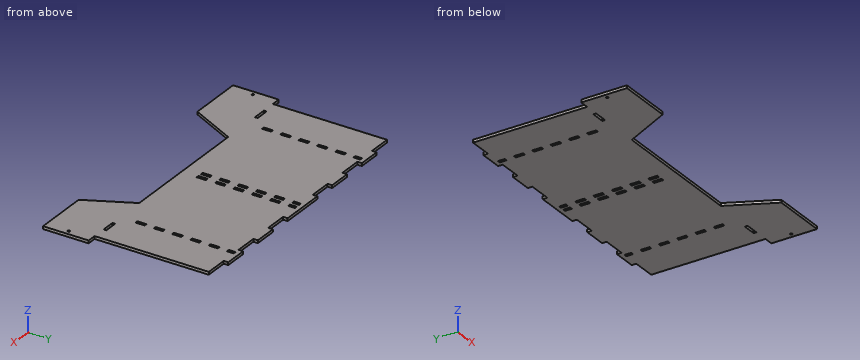
```python
from build123d import *

# Parameters (mm, degrees)
SKETCH_1_W      = 6
SKETCH_1_H      = 15
SKETCH_1_R      = 2.5
SKETCH_1_W_2    = 30
SKETCH_1_H_2    = 6
SKETCH_1_H_3    = 20
EXTRUDE_1_DEPTH = 6


with BuildPart() as part:
    # 草图1 → 凸台-拉伸1 (new body)
    with BuildSketch(Plane.XY):
        Polygon((50, 0), (0, 0), (0, -250), (-20, -250), (-20, -350), (100, -350), (150, -250), (450, -250), (500, -350), (620, -350), (620, -250), (600, -250), (600, 0), (550, 0), (550, 10), (500, 10), (500, 0), (450, 0), (450, 10), (400, 10), (400, 0), (350, 0), (350, 10), (300, 10), (250, 10), (250, 0), (200, 0), (200, 10), (150, 10), (150, 0), (100, 0), (100, 10), (50, 10), align=None)
        with Locations((513, -7.5)):
            Rectangle(SKETCH_1_W, SKETCH_1_H, mode=Mode.SUBTRACT)
        with Locations((-10, -300)):
            Circle(SKETCH_1_R, mode=Mode.SUBTRACT)
        with Locations((45, -247)):
            Rectangle(SKETCH_1_W_2, SKETCH_1_H_2, mode=Mode.SUBTRACT)
        with Locations((87, -205)):
            Rectangle(SKETCH_1_W, SKETCH_1_H_3, mode=Mode.SUBTRACT)
        with Locations((87, -165)):
            Rectangle(SKETCH_1_W, SKETCH_1_H_3, mode=Mode.SUBTRACT)
        with Locations((293, -205)):
            Rectangle(SKETCH_1_W, SKETCH_1_H_3, mode=Mode.SUBTRACT)
        with Locations((293, -165)):
            Rectangle(SKETCH_1_W, SKETCH_1_H_3, mode=Mode.SUBTRACT)
        with Locations((610, -300)):
            Circle(SKETCH_1_R, mode=Mode.SUBTRACT)
        with Locations((555, -247)):
            Rectangle(SKETCH_1_W_2, SKETCH_1_H_2, mode=Mode.SUBTRACT)
        with Locations((307, -205)):
            Rectangle(SKETCH_1_W, SKETCH_1_H_3, mode=Mode.SUBTRACT)
        with Locations((307, -165)):
            Rectangle(SKETCH_1_W, SKETCH_1_H_3, mode=Mode.SUBTRACT)
        with Locations((513, -205)):
            Rectangle(SKETCH_1_W, SKETCH_1_H_3, mode=Mode.SUBTRACT)
        with Locations((513, -165)):
            Rectangle(SKETCH_1_W, SKETCH_1_H_3, mode=Mode.SUBTRACT)
        with Locations((87, -125)):
            Rectangle(SKETCH_1_W, SKETCH_1_H_3, mode=Mode.SUBTRACT)
        with Locations((87, -85)):
            Rectangle(SKETCH_1_W, SKETCH_1_H_3, mode=Mode.SUBTRACT)
        with Locations((293, -125)):
            Rectangle(SKETCH_1_W, SKETCH_1_H_3, mode=Mode.SUBTRACT)
        with Locations((293, -85)):
            Rectangle(SKETCH_1_W, SKETCH_1_H_3, mode=Mode.SUBTRACT)
        with Locations((87, -45)):
            Rectangle(SKETCH_1_W, SKETCH_1_H_3, mode=Mode.SUBTRACT)
        with Locations((87, -7.5)):
            Rectangle(SKETCH_1_W, SKETCH_1_H, mode=Mode.SUBTRACT)
        with Locations((293, -45)):
            Rectangle(SKETCH_1_W, SKETCH_1_H_3, mode=Mode.SUBTRACT)
        with Locations((293, -7.5)):
            Rectangle(SKETCH_1_W, SKETCH_1_H, mode=Mode.SUBTRACT)
        with Locations((307, -125)):
            Rectangle(SKETCH_1_W, SKETCH_1_H_3, mode=Mode.SUBTRACT)
        with Locations((307, -85)):
            Rectangle(SKETCH_1_W, SKETCH_1_H_3, mode=Mode.SUBTRACT)
        with Locations((513, -125)):
            Rectangle(SKETCH_1_W, SKETCH_1_H_3, mode=Mode.SUBTRACT)
        with Locations((513, -85)):
            Rectangle(SKETCH_1_W, SKETCH_1_H_3, mode=Mode.SUBTRACT)
        with Locations((307, -45)):
            Rectangle(SKETCH_1_W, SKETCH_1_H_3, mode=Mode.SUBTRACT)
        with Locations((307, -7.5)):
            Rectangle(SKETCH_1_W, SKETCH_1_H, mode=Mode.SUBTRACT)
        with Locations((513, -45)):
            Rectangle(SKETCH_1_W, SKETCH_1_H_3, mode=Mode.SUBTRACT)
    extrude(amount=EXTRUDE_1_DEPTH)


solid = part.part
```
Model file for the job. Use its own axes, mm. Round coordinates to 2 decimals unless told otherwise and drop trailing zeros. Loops run counter-clockwise (first coordinate to the right, second up) from the corner with the lowest first, then second, coordinate; pieces in that order, holes last. Notation, with made-up numbers: M 29,-27.5 L 69,-27.5 A17 ccw 69,-10.5 Z; hole C -17,57.25 d2. An arc over 180 degrees is marked long. Put each result on its own line as item: value. Start each with the question number.
Item 1: Cut at A-A (y = -224). List the corners of the cut face in (x, z), then the cut area to 3 significant figures.
Item 2: Cut at B-B (x = 114). List the corners of the cut face in (y, z), then the cut area to 3 significant figures.
Item 3: Cut at C-C (z = 3.9). Give the number of separate pieces and of enclosed holes in the cut face, then the cut area to 3 significant figures.
Item 4: Drill centre lines: line 1 along X through (y, z) = (-46.5, 2.65); line 2 along Y through (x, z) = (610, 4.65); line 3 along X through (y, z) = (-300, 3.8). Where is each one in solid material? Low to high.
Item 5: Drop flat-ended pins along their axis: P1, Ø3, axis at y = -204, z = 4.5, coming from the -X side; P2, Ø3, axis at y = 6, z = 2.5, coming from the +X side; P3, Ø1.8, axis at x = 551.5, z = 4, coming from the +Y side. Give the stop position or say it passes through.
Answer block:
1. outline: M 0,0 L 600,0 L 600,6 L 0,6 Z
1. area: 3,600 mm2
2. outline: M -322,0 L 0,0 L 0,6 L -322,6 Z
2. area: 1,930 mm2
3. separate pieces: 1
3. enclosed holes: 28
3. area: 179,000 mm2
4. line 1: 0 to 84, 90 to 290, 296 to 304, 310 to 510, 516 to 600
4. line 2: -350 to -302.5, -297.5 to -250
4. line 3: -20 to -12.5, -7.5 to 125, 475 to 607.5, 612.5 to 620
5. P1: x = 0
5. P2: x = 550
5. P3: y = 0
